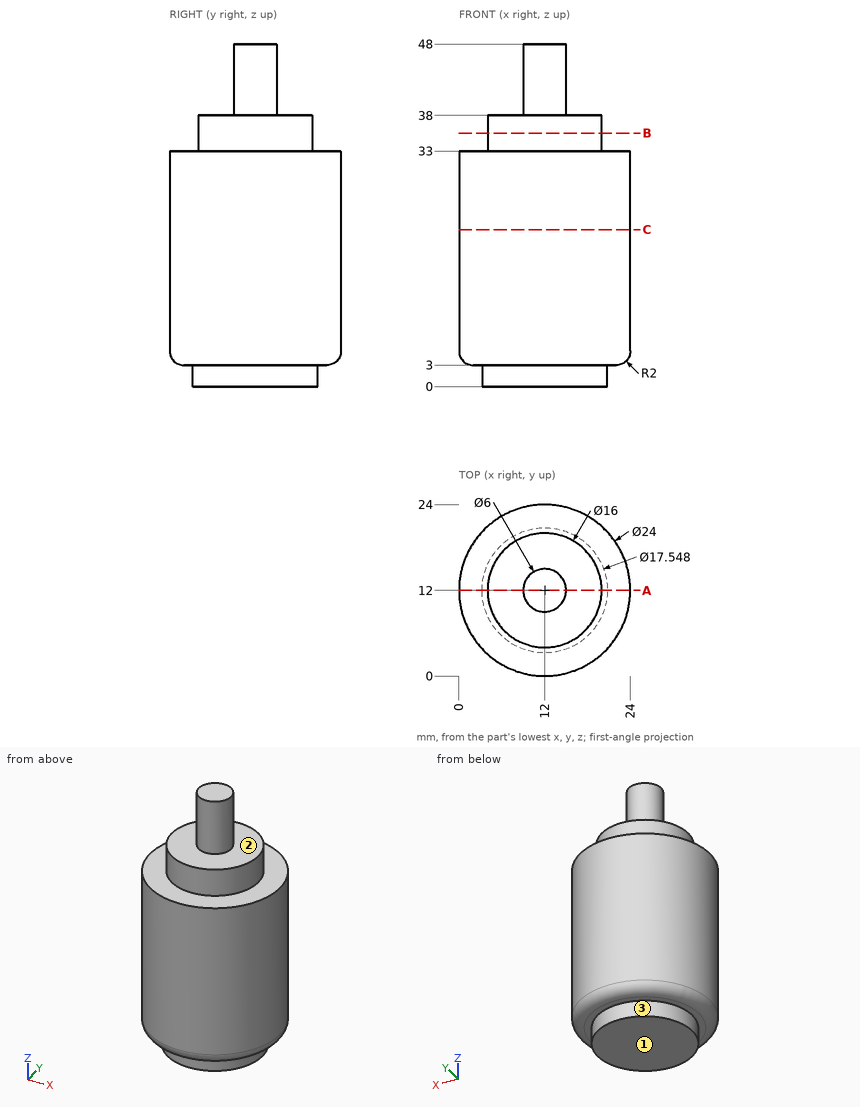
The figure shows three views and two pictorial views of one solid part (mm, origin at its lowest corner). Answer the questions. A direction names the side the tool comes from. Round coordinates to 2 decimals unless told otherwise and drop trailing zeros. Order: outer loops, then holes, each group sorted by start corner. A loop starts at its lowest first (then second) coordinate and runs counter-clockwise, first axis right, second up. Notation, with made-up numbers: M 69.25,64 L 85.25,64 A19 ccw 85.25,88 Z; hole C 82.5,58.5 d2. An arc over 180 degrees is marked long. Put each result on its own line as item: value. Start each with the question number.
Q1. Flat-ended cylindrical pins translate along their axes: pin 1 (6 mm diameter, centred on x = 11.5, z = 42.5, fed in from +Y); pin 2 (4 mm diameter, centred on x = 6, z = 7, fed in from +Y); pin 3 (3 mm diameter, centred on y = 16, z = 31.5, fed in from -X). Find the tip coordinate at first contact, or state that the pin passes through.
Q2. Section C-C, the plane z = 22 is taken. Write down the section's boundary in (x, y), and give its area (3 significant figures).
Q3. Section B-B, the plane z = 35.5 is taken. Write down the section's boundary in (x, y).
Q4. Straight lines are drawn through the part: L1, parallel to Z at x = 9, y = 7; L2, parallel to X at y = 12.25, z = 12.5; L3, parallel to Z at x = 19.75, y = 9.5. For each, find the intervals that lie inside material, in ascending order. Write a range as [from, to].
Q5. Section A-A, the plane y = 12 is taken. Write down the section's boundary in (x, z).
Q6. A tool of negligible diameter and unlimited length cuts with its end or side. For the marked faces 1, 2 and 3, from which of +Z, -Z, +X, -X, +Y, -Y can it reach the whole face along a straight path? Write none if from no direction.
Findings below:
1. pin 1: stops at y = 15
1. pin 2: stops at y = 23.31
1. pin 3: stops at x = 0.26
2. outline: C 12,12 d24
2. area: 452 mm^2
3. outline: C 12,12 d16
4. L1: z = [0, 38]
4. L2: x = [0, 24]
4. L3: z = [0, 33]
5. outline: M 0,5 A2 ccw 2,3 L 3.23,3 L 3.23,0 L 20.77,0 L 20.77,3 L 22,3 A2 ccw 24,5 L 24,33 L 20,33 L 20,38 L 15,38 L 15,48 L 9,48 L 9,38 L 4,38 L 4,33 L 0,33 Z
6. face 1: -Z, +X, -X, +Y, -Y
6. face 2: +Z
6. face 3: -Z
